from build123d import *

# Parameters (mm, degrees)
EXTRUDE_1_DEPTH = 10
EXTRUDE_2_DEPTH = 7


with BuildPart() as part:
    # Эскиз1 → Вытянуть1 (new body)
    with BuildSketch(Plane.XY):
        with BuildLine():
            Line((0.2, 0.695621493), (0.2, 3.304378507))
            ThreePointArc((0.2, 3.304378507), (0.407098908, 3.589631705), (0.74246258, 3.481047398))
            ThreePointArc((0.74246258, 3.481047398), (0.840114832, 2.729978951), (0.260484004, 2.242467025))
            Line((0.260484004, 2.242467025), (0.3, 2.046409671))
            ThreePointArc((0.3, 2.046409671), (1.026500083, 2.657449384), (0.9041043, 3.598826659))
            ThreePointArc((0.9041043, 3.598826659), (0.345164846, 3.779800504), (0, 3.304378507))
            Line((0, 3.304378507), (0, 0.695621493))
            ThreePointArc((0, 0.695621493), (0.345164846, 0.220199496), (0.9041043, 0.401173341))
            ThreePointArc((0.9041043, 0.401173341), (1.026500083, 1.342550616), (0.3, 1.953590329))
            Line((0.3, 1.953590329), (0.260484004, 1.757532975))
            ThreePointArc((0.260484004, 1.757532975), (0.840114832, 1.270021049), (0.74246258, 0.518952602))
            ThreePointArc((0.74246258, 0.518952602), (0.407098908, 0.410368295), (0.2, 0.695621493))
        make_face()
    extrude(amount=EXTRUDE_1_DEPTH)

    # Эскиз2 → Вытянуть2 (add)
    with BuildSketch(Plane(origin=(0, 0, 0), x_dir=(-1, 0, 0), z_dir=(0, 0, -1))):
        with BuildLine():
            Line((-2.490967365, 1.85), (-2.289230485, 1.85))
            ThreePointArc((-2.289230485, 1.85), (-0.2, 2), (-2.289230485, 2.15))
            Line((-2.289230485, 2.15), (-2.490967365, 2.15))
            ThreePointArc((-2.490967365, 2.15), (0, 2), (-2.490967365, 1.85))
        make_face()
    extrude(amount=EXTRUDE_2_DEPTH)


solid = part.part
Geometry check sheet. Reference: the model listing, model coordinates, mm. A direction names the side the tool comes from. Give positions to 0.01 mm unless a question says otherwise; leave off trailing zeros. Loops run counter-clockwise (first coordinate to the right, second up) from the corner with the lowest first, then second, coordinate; pieces in that order, holes last.
(1) Depth check by flat-ended pin: pin 1 Ø1.2 at (x, y) = (2, 1.5) entering from +Z; pin 2 Ø1.3 at (y, z) = (2, 6) entering from +X. Enter the tip coordinate at first touch or a pass-through.
From the geometry:
pin 1: stops at z = 0
pin 2: stops at x = 1.02
(2) Section check A-A on x = 1.25. Record the cut outline in (y, z), then the cut area to 3 significant figures.
From the geometry:
outline: (0.75, -7) - (0.95, -7) - (0.95, 0) - (0.75, 0) - close; (3.05, -7) - (3.25, -7) - (3.25, 0) - (3.05, 0) - close
area: 2.80 mm2
(3) Release check for a two-part mould opening along Y. For faces 1 (the cylindrical face through (0, 2, -3)), 2 (the flat face through (0, 2, 5)), 3 (the cylindrical face through (0.35, 3.78, 4.93)), 4 (the cylindrical face through (1, 2.6, 4.9)) record: released by +Y, released by -Y, zero draft, split by the parting line, or undercut.
From the geometry:
face 1: split by the parting line
face 2: zero draft
face 3: released by +Y
face 4: undercut
(4) Section check B-B on z = 8.25. Record the cut outline in (x, y), then the cut area to 3 significant figures.
From the geometry:
outline: (0, 0.7) arc R0.5 ccw to (0.9, 0.4) arc R0.99 ccw to (0.3, 1.95) - (0.26, 1.76) arc R0.79 cw to (0.74, 0.52) arc R0.3 cw to (0.2, 0.7) - (0.2, 3.3) arc R0.3 cw to (0.74, 3.48) arc R0.79 cw to (0.26, 2.24) - (0.3, 2.05) arc R0.99 ccw to (0.9, 3.6) arc R0.5 ccw to (0, 3.3) - close
area: 1.64 mm2
(5) Thickness scan on L1, parallel to Y at x = 1.25, z = -4.75; L2, parallel to Y at x = 0.8, z = 7; L3, parallel to X at y = 2, z = -2.5. Record the ranges inside material, lowest first.
From the geometry:
L1: y = 0.75 to 0.95, 3.05 to 3.25
L2: y = 0.3 to 0.61, 1.36 to 1.69, 2.31 to 2.64, 3.39 to 3.7
L3: x = 0 to 0.2
(6) Set-up check for faces 5 (the cylindrical face through (0.34, 0.22, 4.93)), 6 (the cylindrical face through (0.2, 2, -3.5)), 7 (the flat face through (0.2, 3, 5)): record each of +Z, -Z, +X, -X, +Y, -Y from which the full face is reachable in a straight line by a thin tool's end or side.
From the geometry:
face 5: +Z, -Z, -Y
face 6: -Z
face 7: +Z
(7) Section check C-C on x = 2.1. Record the cut outline in (y, z), then the cut area to 3 significant figures.
From the geometry:
outline: (1.08, -7) - (1.38, -7) - (1.38, 0) - (1.08, 0) - close; (2.62, -7) - (2.92, -7) - (2.92, 0) - (2.62, 0) - close
area: 4.20 mm2
(8) Section check D-D on z = -0.75. Record the cut outline in (x, y), then the cut area to 3 significant figures.
From the geometry:
outline: (2.29, 1.85) arc R1.05 cw (long way) to (2.29, 2.15) - (2.49, 2.15) arc R1.25 ccw (long way) to (2.49, 1.85) - close
area: 1.38 mm2
